Part model, mm, in its own coordinate system. Round coordinates to 2 decimals unless told otherwise and drop trailing zeros. Write each loop counter-clockwise with the first axis right and the second up, starting at its lowest first coordinate (ties: lowest second). Pieces come first, ordered by that corner, then holes. Notation, with made-up numbers: M 87,70.25 L 145,70.25 A36 cw 145,106.25 Z; hole C 70.5,19.25 d2. An arc over 180 degrees is marked long. Answer as a JSON object with one key per item and string values. Group by question number.
1. Drill centre lines: line 1 (Y direction, x = -12.5, z = 2.1); line 2 (X direction, y = 2, z = 1.25); line 3 (Y direction, x = -86, z = 0.75). Where is each one in solid material? Low to high. Write a range as from..to.
2. Band-saw the part on B-B, the plane y = 84. Write the cut outline in (x, z).
3. Band-saw the part on A-A, the plane z = 1.05. Count the separate pieces of the cut face and the enclosed holes in it, plus the area to 3 significant figures.
4. Band-saw the part on C-C, the plane x = 34. Write the cut outline in (y, z), plus the area to 3 significant figures.
5. Drop flat-ended pins along their axis: pin 1 (1.5 mm diameter, centred on x = -115.5, z = 2, fed in from +Y); pin 2 (1 mm diameter, centred on x = -62, z = 1.5, fed in from -Y); pin 3 (1.8 mm diameter, centred on x = 13.64, y = -20.95, fed in from +Z); pin 4 (1.5 mm diameter, centred on y = 80.5, z = 1, fed in from -X). Give the stop position or say it passes through.
from build123d import *

# Parameters (mm, degrees)
SKETCH1_R                       = 150
SKETCH1_R_2                     = 2.4
BOSS_EXTRUDE2_DEPTH             = 3
F_3_0MM_DOWEL_HOLE2_D           = 3
F_3_0MM_DOWEL_HOLE2_CSINK_D     = 3.05
F_3_0MM_DOWEL_HOLE2_CSINK_ANGLE = 90


with BuildPart() as part:
    # Sketch1 → Boss-Extrude2 (new body)
    with BuildSketch(Plane.XY):
        Circle(SKETCH1_R)
        with Locations((12.5, 140)):
            Circle(SKETCH1_R_2, mode=Mode.SUBTRACT)
        with Locations((-12.5, 140)):
            Circle(SKETCH1_R_2, mode=Mode.SUBTRACT)
        with Locations((127.49355653, -59.174682453)):
            Circle(SKETCH1_R_2, mode=Mode.SUBTRACT)
        with Locations((114.99355653, -80.825317547)):
            Circle(SKETCH1_R_2, mode=Mode.SUBTRACT)
        with Locations((-114.99355653, -80.825317547)):
            Circle(SKETCH1_R_2, mode=Mode.SUBTRACT)
        with Locations((-127.49355653, -59.174682453)):
            Circle(SKETCH1_R_2, mode=Mode.SUBTRACT)
    extrude(amount=BOSS_EXTRUDE2_DEPTH)

    # Ø3.0mm Dowel Hole2 (through all)
    with Locations(Plane(origin=(0, 0, 0), x_dir=(-1, 0, 0), z_dir=(0, 0, -1))):
        with Locations((-20.948618644, 13.643876902), (13.643876902, 20.948618644), (20.948618644, -13.643876902), (-13.643876902, -20.948618644)):
            CounterSinkHole(F_3_0MM_DOWEL_HOLE2_D / 2, F_3_0MM_DOWEL_HOLE2_CSINK_D / 2, counter_sink_angle=F_3_0MM_DOWEL_HOLE2_CSINK_ANGLE)


solid = part.part
Worked answers:
{
 "1": {"line 1": "y = -149.48..19.98, 21.92..137.6, 142.4..149.48", "line 2": "x = -149.99..149.99", "line 3": "y = -122.9..122.9"},
 "2": {"outline": "M -124.27,0 L 124.27,0 L 124.27,3 L -124.27,3 Z"},
 "3": {"separate pieces": "1", "enclosed holes": "10", "area": "70,500 mm^2"},
 "4": {"outline": "M -146.1,0 L 146.1,0 L 146.1,3 L -146.1,3 Z", "area": "877 mm^2"},
 "5": {"pin 1": "stops at y = 96.6", "pin 2": "stops at y = -136.81", "pin 3": "passes through", "pin 4": "stops at x = -127.04"}
}
